```python
from build123d import *

# Parameters (mm, degrees)
SKETCH1_W           = 6.35
SKETCH1_H           = 43.18
BOSS_EXTRUDE1_DEPTH = 288.29
CUT_EXTRUDE1_REACH  = 293.575
SKETCH2_W           = 50.8
SKETCH2_H           = 12.7


with BuildPart() as part:
    # Sketch1 → Boss-Extrude1 (new body)
    with BuildSketch(Plane.XY):
        with Locations((3.175, 21.59)):
            Rectangle(SKETCH1_W, SKETCH1_H)
    extrude(amount=BOSS_EXTRUDE1_DEPTH)

    # Sketch2 → Cut-Extrude1 (cut, up to next)
    with BuildSketch(Plane.ZY, mode=Mode.PRIVATE) as cut_extrude1_sk1:
        with Locations((262.89, 6.35)):
            Rectangle(SKETCH2_W, SKETCH2_H)
    cut_extrude1_tool1 = extrude(cut_extrude1_sk1.sketch, amount=-CUT_EXTRUDE1_REACH, mode=Mode.PRIVATE) & part.part
    add(cut_extrude1_tool1.solids().sort_by_distance((0, 6.35, 262.89))[0], mode=Mode.SUBTRACT)


solid = part.part
```
Input: part model. Units: mm. Frame: model coordinates. A direction names the side the tool comes from. Round coordinates to 2 decimals unless told otherwise and drop trailing zeros. Loops run counter-clockwise (first coordinate to the right, second up) from the corner with the lowest first, then second, coordinate; pieces in that order, holes last. Notation, with made-up numbers: (62.5, 68.25) -> (106.5, 68.25) arc R12 cw to (106.5, 87.25) -> close; hole circle Ø3 at (9.25, 75.25). An arc over 180 degrees is marked (long way). Use one line per item in the form item = value. Start each with the question number.
Item 1: Contact query for flat-ended pins moving along their axis: pin 1 Ø1.9 at (x, y) = (2, 9.5) entering from +Z; pin 2 Ø3 at (x, z) = (4, 265) entering from -Y. Output: stop coordinate, or through.
Item 2: Material intervals for L1, parallel to Z at x = 5.25, y = 11.5; L2, parallel to Y at x = 1.5, z = 245.5, sorted ascending. Write a range as from..to.
Item 3: Set-up query: faces 1 (the face through (3, 12.7, 263)), 2 (the face through (3, 22, 0)). Return all of +Z, -Z, +X, -X, +Y, -Y with unobstructed straight access to the full face (end or side cutting, diameter ignored); none if empty.
Item 4: Section query A-A on x = 4.5. Return the cut outline in (y, z), then the cut area to 3 significant figures.
Ans:
q1.pin_1 = 237.49
q1.pin_2 = 12.7
q2.L1 = 0..237.49
q2.L2 = 12.7..43.18
q3.face_1 = +Z, +X, -X, -Y
q3.face_2 = -Z, +X, -X, +Y, -Y
q4.outline = (0, 0) -> (43.18, 0) -> (43.18, 288.29) -> (12.7, 288.29) -> (12.7, 237.49) -> (0, 237.49) -> close
q4.area = 11,800 mm^2
